Check sheet for the drawn part. Datum: minimum x, y, z corner. Units: mm. A direction names the side the tool comes from. Coordinates: 2 decimals unless noted, no trailing zeros. Loops run counter-clockwise (first coordinate to the right, second up) from the corner with the lowest first, then second, coordinate; pieces in that order, holes last. Notation, with made-up numbers: (54, 65) - (78, 65) arc R20 ccw to (78, 96) - close; hole circle Ø10 at (34, 31.5). An arc over 180 degrees is marked (long way). Answer as CSV lines item,"result". Start each with the question number.
1. Set-up check for the marked faces 1 and 2: record each of +Z, -Z, +X, -X, +Y, -Y from which the full face is reachable in a straight line by a thin tool's end or side.
2. Cross-section at D-D (y = 31). Enter the section's corners in (x, z).
3. Material ranges on line 1 (Y direction, x = 35, z = 66); line 2 (Y direction, x = 67.5, z = 12); line 3 (Y direction, x = 60, z = 68), recorded low to high. Write a range as [from, to].
4. Gauge pin test, flat ends, axial feed: P1, Ø8, axis at x = 44.5, y = 35.5, coming from the +Z side; P2, Ø6.5, axis at y = 58, z = 58, coming from the -X side; P3, Ø8, axis at x = 60, y = 35, coming from the -Z side. Record the tip position at first contact, or that the pin passes through.
5. Cross-section at B-B (x = 35). Enter the section's corners in (y, z), plus the area to 3 significant figures.
6. Cross-section at A-A (z = 12). Enter the section's corners in (x, y), plus the area to 3 significant figures.
7. Cross-section at C-C (x = 60). Enter the section's corners in (y, z).
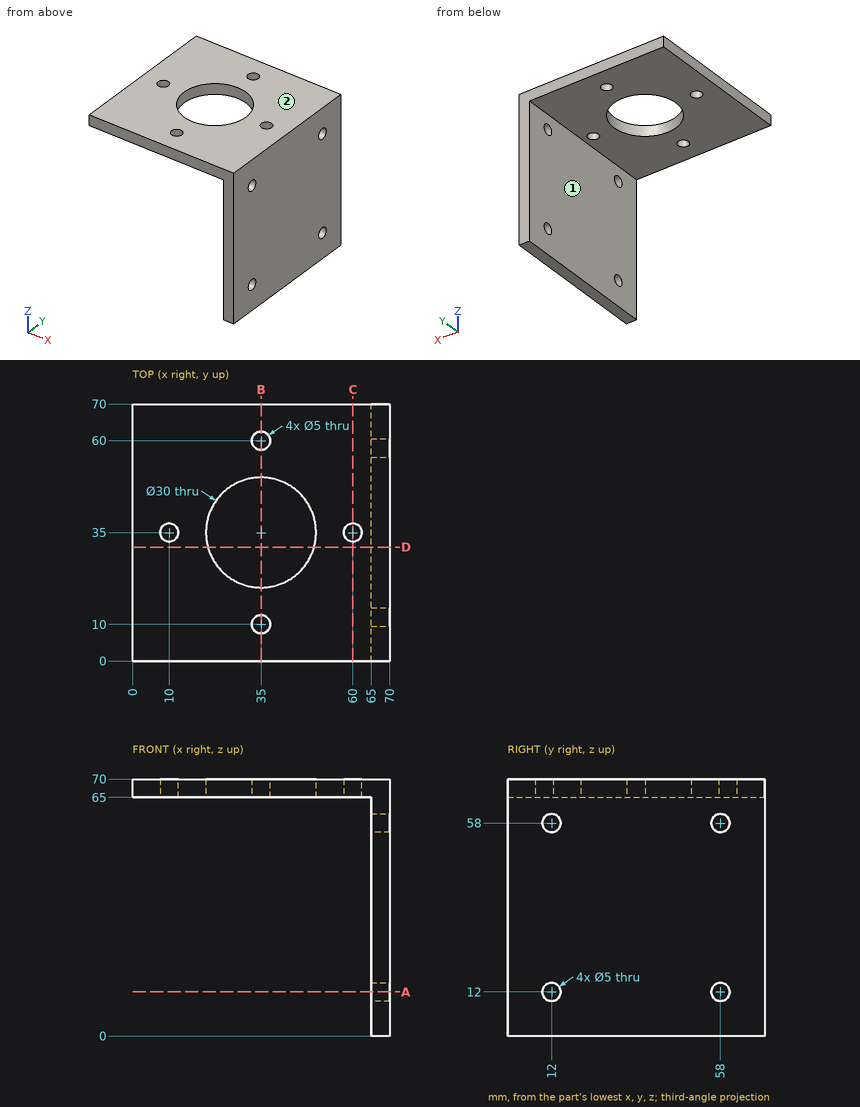
Values follow:
1,face 1,"-Z, -X, +Y, -Y"
1,face 2,"+Z, +X, -X, +Y, -Y"
2,outline,"(0, 65) - (20.54, 65) - (20.54, 70) - (0, 70) - close; (49.46, 65) - (65, 65) - (65, 0) - (70, 0) - (70, 70) - (49.46, 70) - close"
3,line 1,"y = [0, 7.5], [12.5, 20], [50, 57.5], [62.5, 70]"
3,line 2,"y = [0, 9.5], [14.5, 55.5], [60.5, 70]"
3,line 3,"y = [0, 32.5], [37.5, 70]"
4,P1,"passes through"
4,P2,"stops at x = 65"
4,P3,"stops at z = 65"
5,outline,"(0, 65) - (7.5, 65) - (7.5, 70) - (0, 70) - close; (12.5, 65) - (20, 65) - (20, 70) - (12.5, 70) - close; (50, 65) - (57.5, 65) - (57.5, 70) - (50, 70) - close; (62.5, 65) - (70, 65) - (70, 70) - (62.5, 70) - close"
5,area,"150 mm²"
6,outline,"(65, 0) - (70, 0) - (70, 9.5) - (65, 9.5) - close; (65, 14.5) - (70, 14.5) - (70, 55.5) - (65, 55.5) - close; (65, 60.5) - (70, 60.5) - (70, 70) - (65, 70) - close"
6,area,"300 mm²"
7,outline,"(0, 65) - (32.5, 65) - (32.5, 70) - (0, 70) - close; (37.5, 65) - (70, 65) - (70, 70) - (37.5, 70) - close"
